Part model, mm, in its own coordinate system. Round coordinates to 2 decimals unless told otherwise and drop trailing zeros. Loops run counter-clockwise (first coordinate to the right, second up) from the corner with the lowest first, then second, coordinate; pieces in that order, holes last.
1) Band-saw the part on A-A, the plane x = 0. Write the cut outline in (y, z), then the cut area to 3 significant figures.
2) Drop a flat-ended pin along its axis: P1, Ø1, axis at y = -0.5, z = 1.5, coming from the -X side. Give the stop position or say it passes through.
3) Band-saw the part on C-C, the plane y = -5.25. Write the cut outline in (x, z), then the cut area to 3 significant figures.
4) Probe line 1 (Z direction, x = 0.1, y = -1.75); line 2 (Y direction, x = 0, z = 4). List the from-to ranges inside material, lowest first.
5) Band-saw the part on B-B, the plane z = 5.25. Write the cut outline in (x, y).
from build123d import *
from OCP.BRepFilletAPI import BRepFilletAPI_MakeChamfer

# Parameters (mm, degrees)
ESBO_O2_W      = 0.5
ESBO_O2_H      = 0.5
CHANFRO1_SIZE  = 0.1
CHANFRO1_SIZE2 = 0.3
CHANFRO2_SIZE  = 0.3
CHANFRO2_SIZE2 = 0.1


with BuildPart() as part:
    # Varredura1: sweep along a path in Esboço1
    with BuildLine(Plane(origin=(0, 0, 0), x_dir=(0, 0, -1), z_dir=(1, 0, 0))) as varredura1_path:
        Line((0, 0), (-5.5, 0))
        ThreePointArc((-5.5, 0), (-5.853553391, -0.146446609), (-6, -0.5))
        Line((-6, -0.5), (-6, -6))
    # Esboço2 → Varredura1 (sweep)
    with BuildSketch(Plane.XY):
        Rectangle(ESBO_O2_W, ESBO_O2_H)
    sweep(path=varredura1_path.line)

    # Chanfro1
    chanfro1_edges = [part.edges().sort_by_distance(p)[0] for p in [
        (0, 0.25, 0),
        (-0.25, 0, 0),
        (0, -0.25, 0),
        (0.25, 0, 0),
    ]]
    chanfro1_side = [part.faces().sort_by_distance(p)[0] for p in [
        (0, 0, 0),
    ]]
    chamfer(chanfro1_edges, length=CHANFRO1_SIZE, length2=CHANFRO1_SIZE2, reference=chanfro1_side[0])

    # Chanfro2: one chamfer whose edges measure the first distance from different faces: ONE call of the kernel's chamfer builder (chamfer() names one face for all edges)
    chanfro2_edges_1 = [part.edges().sort_by_distance(p)[0] for p in [
        (0.25, -6, 6),
    ]]
    chanfro2_side_1 = [part.faces().sort_by_distance(p)[0] for p in [
        (0.25, -0.163706895, 2.9),
    ]]
    chanfro2_edges_2 = [part.edges().sort_by_distance(p)[0] for p in [
        (0, -6, 6.25),
    ]]
    chanfro2_side_2 = [part.faces().sort_by_distance(p)[0] for p in [
        (0, -3.25, 6.25),
    ]]
    chanfro2_edges_3 = [part.edges().sort_by_distance(p)[0] for p in [
        (-0.25, -6, 6),
    ]]
    chanfro2_side_3 = [part.faces().sort_by_distance(p)[0] for p in [
        (-0.25, 0.163706895, 2.9),
    ]]
    chanfro2_edges_4 = [part.edges().sort_by_distance(p)[0] for p in [
        (0, -6, 5.75),
    ]]
    chanfro2_side_4 = [part.faces().sort_by_distance(p)[0] for p in [
        (0, -3.25, 5.75),
    ]]
    chanfro2 = BRepFilletAPI_MakeChamfer(part.part.solid().wrapped)
    for e in chanfro2_edges_1:
        chanfro2.Add(CHANFRO2_SIZE, CHANFRO2_SIZE2, e.wrapped, chanfro2_side_1[0].wrapped)  # the first distance lies on this face
    for e in chanfro2_edges_2:
        chanfro2.Add(CHANFRO2_SIZE, CHANFRO2_SIZE2, e.wrapped, chanfro2_side_2[0].wrapped)  # the first distance lies on this face
    for e in chanfro2_edges_3:
        chanfro2.Add(CHANFRO2_SIZE, CHANFRO2_SIZE2, e.wrapped, chanfro2_side_3[0].wrapped)  # the first distance lies on this face
    for e in chanfro2_edges_4:
        chanfro2.Add(CHANFRO2_SIZE, CHANFRO2_SIZE2, e.wrapped, chanfro2_side_4[0].wrapped)  # the first distance lies on this face
    add(Compound.cast(chanfro2.Shape()), mode=Mode.REPLACE)


solid = part.part
Reported:
1. outline: (-6, 5.85) - (-5.7, 5.75) - (-0.5, 5.75) arc R0.25 cw to (-0.25, 5.5) - (-0.25, 0.3) - (-0.15, 0) - (0.15, 0) - (0.25, 0.3) - (0.25, 5.5) arc R0.75 ccw to (-0.5, 6.25) - (-5.7, 6.25) - (-6, 6.15) - close
1. area: 5.83 mm2
2. P1: stops at x = -0.25
3. outline: (-0.25, 5.75) - (0.25, 5.75) - (0.25, 6.25) - (-0.25, 6.25) - close
3. area: 0.250 mm2
4. line 1: z = 5.75 to 6.25
4. line 2: y = -0.25 to 0.25
5. outline: (-0.25, -0.25) - (0.25, -0.25) - (0.25, 0.25) - (-0.25, 0.25) - close
